Source: CAD feature listing. Evaluate the final solid. Frame: model axes, mm. Give positions to 0.01 mm unless a question says otherwise; leave off trailing zeros. Order: outer loops, then holes, each group sorted by start corner. A loop starts at its lowest first (then second) coordinate and runs counter-clockwise, first axis right, second up. Notation, with made-up numbers: (8.5, 69.25) -> (60.5, 69.25) arc R23 cw to (60.5, 98.25) -> close; hole circle Ø6 at (-39.5, -34.5). An arc over 180 degrees is marked (long way). Use CSV: the item, a comma, the result in double quotes.
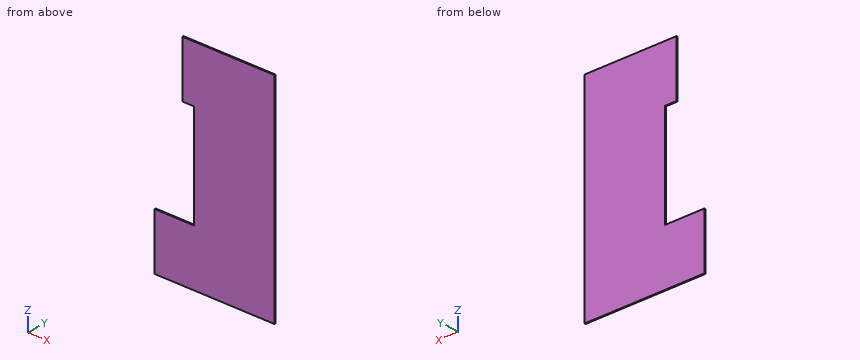
Autodesk Inventor part; units mm, degrees
ref_plane "YZ Plane" through (0, 0, 0) normal (1, 0, 0) x (0, 1, 0)
ref_plane "XZ Plane" through (0, 0, 0) normal (0, 1, 0) x (-1, 0, 0)
ref_plane "XY Plane" through (0, 0, 0) normal (0, 0, 1) x (1, 0, 0)
sketch "Sketch1" plane through (0, 0, 0) normal (0, 0, 1) x (1, 0, 0)
  line L0 (0, 0) -> (254, 0)
  line L1 (254, 0) -> (254, 3.175)
  line L2 (254, 3.175) -> (0, 3.175)
  line L3 (0, 3.175) -> (0, 0)
  dimension "d0" = 254
  dimension "d1" = 3.175
extrude "Extrusion1" add sketch "Sketch1" along normal blind 584.2
sketch "Sketch2" plane through (0, 3.175, 0) normal (0, 1, 0) x (1, 0, 0)
  line L0 (0, -584.2) -> (254, -584.2)
  line L1 (254, 0) -> (0, 0)
  line L2 (0, 0) -> (0, -584.2)
  line L3 (0, -152.4) -> (31.75, -152.4)
  line L4 (31.75, -152.4) -> (31.75, -431.8)
  line L5 (31.75, -431.8) -> (0, -431.8)
  line L6 (0, -431.8) -> (0, -152.4)
  line L7 (31.75, -152.4) -> (31.75, 0) construction
  line L8 (31.75, -431.8) -> (31.75, -584.2) construction
  dimension "d4" = 31.75
  dimension "d5" = 279.4
extrude "Extrusion2" cut sketch "Sketch2" against normal through all
sketch "Sketch3" plane through (0, 0, 0) normal (-1, 0, 0) x (0, 0, 1)
  line L0 (0, 0) -> (152.4, 0)
  line L1 (152.4, 0) -> (152.4, 3.175)
  line L2 (152.4, 3.175) -> (0, 3.175)
  line L3 (0, 3.175) -> (0, 0)
extrude "Extrusion3" add sketch "Sketch3" along normal blind 76.2
properties part number "Board_V1" material "ABS Plastic"
1. Ray query, line 1 along Z through (x, y) = (-2.5, 0.7); line 2 along X through (y, z) = (2.3, 243); line 3 along X through (y, z) = (1.8, 547). Return the intervals inside material, ascending.
Answer below:
line 1,"z = 0 to 152.4"
line 2,"x = 31.75 to 254"
line 3,"x = 0 to 254"
2. Section query B-B on x = -12.5. Return loops of the section in (y, z) (3 decimals), plus the area to 3 significant figures.
Answer below:
outline,"(0, 0) -> (3.175, 0) -> (3.175, 152.4) -> (0, 152.4) -> close"
area,"484 mm²"
3. Section query C-C on z = 339. Return loops of the section in (x, y) (3 decimals).
Answer below:
outline,"(31.75, 0) -> (254, 0) -> (254, 3.175) -> (31.75, 3.175) -> close"
4. Section query A-A on y = 1.4. Return loops of the section in (x, z), plus the area to 3 significant figures.
Answer below:
outline,"(-76.2, 0) -> (254, 0) -> (254, 584.2) -> (0, 584.2) -> (0, 431.8) -> (31.75, 431.8) -> (31.75, 152.4) -> (-76.2, 152.4) -> close"
area,"151,000 mm²"
5. Pin query (flat end, axial travel): P1, Ø1, axis at y = 1.5, z = 502.5, coming from the -X side. Return the tip coordinate at first contact, or that it passes through.
Answer below:
P1,"stops at x = 0"
